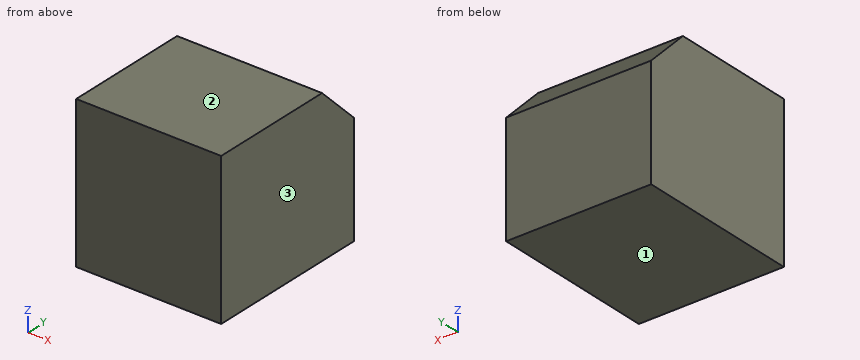
from build123d import *

# Parameters (mm, degrees)
SKETCH1_W           = 29
SKETCH1_H           = 33.4
BOSS_EXTRUDE2_DEPTH = 30.3
CUT_EXTRUDE1_DEPTH  = 54.615762608


with BuildPart() as part:
    # Sketch1 → Boss-Extrude2 (new body)
    with BuildSketch(Plane.XY):
        with Locations((14.5, 16.7)):
            Rectangle(SKETCH1_W, SKETCH1_H)
    extrude(amount=BOSS_EXTRUDE2_DEPTH)

    # Sketch2 → Cut-Extrude1 (cut, through all)
    with BuildSketch(Plane.ZY):
        Polygon((22.3, 33.4), (30.3, 25.4), (30.3, 33.4), align=None)
    extrude(amount=-CUT_EXTRUDE1_DEPTH, mode=Mode.SUBTRACT)


solid = part.part
Check sheet for the modelled part. Datum: model origin and axes. Units: mm. Face numbers are marked on the shaded views. Round coordinates to 2 decimals unless told otherwise and drop trailing zeros. Order: outer loops, then holes, each group sorted by start corner. A loop starts at its lowest first (then second) coordinate and runs counter-clockwise, first axis right, second up.
Q1. Scan lines: L1, parallel to Z at x = 6.5, y = 26; L2, parallel to Z at x = 6, y = 31. Record each from-to range of solid material in increasing order.
Filled sheet:
L1: z = 0 to 29.7
L2: z = 0 to 24.7
Q2. Depth check by flat-ended pin: P1, Ø4, axis at x = 6.5, z = 11, coming from the -Y side. Enter the tip coordinate at first touch or a pass-through.
Filled sheet:
P1: stops at y = 0
Q3. Cross-section at A-A, the plane x = 21.5. Enter the section's corners in (y, z), plus the area to 3 significant figures.
Filled sheet:
outline: (0, 0) - (33.4, 0) - (33.4, 22.3) - (25.4, 30.3) - (0, 30.3) - close
area: 980 mm2
Q4. Cross-section at B-B, the plane y = 31. Enter the section's corners in (x, z), plus the area to 3 significant figures.
Filled sheet:
outline: (0, 0) - (29, 0) - (29, 24.7) - (0, 24.7) - close
area: 716 mm2
Q5. Draft check along Z on the marked faces 1, 2 and 3. Enter one of: pulls with the +Z half, pulls with the -Z half, needs draft (parallel to the pull), parting line crosses it, or undercut.
Filled sheet:
face 1: pulls with the -Z half
face 2: pulls with the +Z half
face 3: needs draft
